Part model, mm, in its own coordinate system. A direction names the side the tool comes from. Coordinates: 2 decimals unless noted, no trailing zeros. Loops run counter-clockwise (first coordinate to the right, second up) from the corner with the lowest first, then second, coordinate; pieces in that order, holes last. Notation, with made-up numbers: (80.5, 9) -> (119.5, 9) arc R17 cw to (119.5, 34) -> close; hole circle Ø11 at (46.25, -7.75). An arc over 180 degrees is marked (long way). Use one line per item in the form item = value. Start each with the question number.
(1) Band-saw the part on D-D on z = 15. Give the cut face in (x, y).
(2) Drill centre lines: L1, parallel to X at y = 5.5, z = 0; L2, parallel to X at y = -0.8, z = 0 (3 decimals); L3, parallel to Y at x = 0, z = -6.5. Where is each one in solid material? Low to high. Write a range as [from, to].
(3) Band-saw the part on C-C on y = 1.75. Give the cut face in (x, z), then the cut area to 3 significant figures.
(4) Pin check, flat tips, straight feed: P1, Ø6, axis at x = -15, z = 7, coming from the +Y side; P2, Ø6, axis at x = 0, z = 0, coming from the -Y side; P3, Ø3.5, axis at x = 0, z = 0, coming from the +Y side; P4, Ø3, axis at y = 0, z = 11, coming from the +X side. Stop position of each tip, or through.
(5) 3-axis set-ups, long thin cutter, end or side, ignore diameter. For faces 4 (the flat face through (-4, 1, 0)), 5 (the cylindrical face through (18.23, 5.227, -5.387)), 6 (the flat face through (1.5, 0, -0.7)): which of +Z, -Z, +X, -X, +Y, -Y reach the whole face in a straight line?
(6) Mould opens along Z. For faces 1 (the flat face through (-18, 9, 0)), 2 (the cylindrical face through (0.45, 0.49, -1.43)), 3 (the cylindrical face through (-1.352, -1.972, 4.292)) say: +Z half, -Z half, draft (parallel to the pull), parting line (faces both ways), or undercut.
(7) Band-saw the part on B-B on x = 0. Give the cut face in (y, z) (3 decimals), then the cut area to 3 significant figures.
(8) Band-saw the part on A-A on z = 0. Give the cut face in (x, y) (3 decimals), then the cut area to 3 significant figures.
```python
from build123d import *

# Parameters (mm, degrees)
SKETCH1_R           = 20.25
BOSS_EXTRUDE1_DEPTH = 9
SKETCH2_R           = 17.75
CUT_EXTRUDE1_DEPTH  = 8
CIRPATTERN1_COUNT   = 3
SKETCH5_R           = 1.5
CUT_EXTRUDE2_DEPTH  = 8
CIRPATTERN2_COUNT   = 3
SKETCH7_R           = 4.5
BOSS_EXTRUDE3_DEPTH = 4
SKETCH8_R           = 3.265
CUT_EXTRUDE3_DEPTH  = 4


with BuildPart() as part:
    # Sketch1 → Boss-Extrude1 (new body)
    with BuildSketch(Plane(origin=(0, 0, 0), x_dir=(1, 0, 0), z_dir=(0, 1, 0))):
        with Locations(Location((0, 0, 0), (0, 0, 270))):
            Circle(SKETCH1_R)
    extrude(amount=BOSS_EXTRUDE1_DEPTH)

    # Sketch2 → Cut-Extrude1 (cut)
    with BuildSketch(Plane(origin=(0, 9, 0), x_dir=(1, 0, 0), z_dir=(0, 1, 0))):
        with Locations(Location((0, 0, 0), (0, 0, 270))):
            Circle(SKETCH2_R)
    extrude(amount=-CUT_EXTRUDE1_DEPTH, mode=Mode.SUBTRACT)

    # Sketch4 → CSK SLOT for M2 Countersunk Flat Head Screw1 (revolve, cut)
    with BuildSketch(Plane(origin=(11.609715894, 0, 11.00974554), x_dir=(0, 0, -1), z_dir=(1, 0, 0))):
        Polygon((0, 0), (0, 6.521032743), (1.2, 5.8), (1.2, 1), (2.2, 0), align=None)
    csk_slot_for_m2_countersunk_flat_head_sc = revolve(axis=Axis((11.609715894, -6.35, 11.00974554), (0, 1, 0)), mode=Mode.SUBTRACT)

    # CirPattern1: CSK SLOT for M2 Countersunk Flat Head Screw1 ×3 about axis
    cirpattern1_axis = Axis((0, 0, 0), (0, 1, 0))
    for i in range(1, CIRPATTERN1_COUNT):
        add(csk_slot_for_m2_countersunk_flat_head_sc.rotate(cirpattern1_axis, i * 360 / CIRPATTERN1_COUNT), mode=Mode.SUBTRACT)

    # Sketch5 → Cut-Extrude2 (cut)
    with BuildSketch(Plane.XZ):
        with Locations(Location((0, 0, 0), (0, 0, 270))):
            Circle(SKETCH5_R)
    extrude(amount=-CUT_EXTRUDE2_DEPTH, mode=Mode.SUBTRACT)

    # Sketch6 → M2 Tapped Hole1 (revolve, cut)
    with BuildSketch(Plane(origin=(-4.560794248, 4.445790719, 19.729715047), x_dir=(0.974306915892993, 0, 0.22522440729877435), z_dir=(0, 1, 0))):
        Polygon((0, 0), (0, 4.980688495), (0.8, 4.5), (0.8, 0), align=None)
    m2_tapped_hole1 = revolve(axis=Axis((-5.990969234, 4.445790719, 25.916563963), (0.22522440729877433, 0, -0.9743069158929931)), mode=Mode.SUBTRACT)

    # CirPattern2: M2 Tapped Hole1 ×3 about axis
    cirpattern2_axis = Axis((0, 9, 0), (0, -1, 0))
    for i in range(1, CIRPATTERN2_COUNT):
        add(m2_tapped_hole1.rotate(cirpattern2_axis, i * 360 / CIRPATTERN2_COUNT), mode=Mode.SUBTRACT)

    # Sketch7 → Boss-Extrude3 (add)
    with BuildSketch(Plane.XZ):
        with Locations(Location((0, 0, 0), (0, 0, 90))):
            Circle(SKETCH7_R)
    extrude(amount=BOSS_EXTRUDE3_DEPTH)

    # Sketch8 → Cut-Extrude3 (cut)
    with BuildSketch(Plane.XZ.offset(4)):
        with Locations(Location((0, 0, 0), (0, 0, 270))):
            Circle(SKETCH8_R)
    extrude(amount=-CUT_EXTRUDE3_DEPTH, mode=Mode.SUBTRACT)


solid = part.part
```
A:
q1.outline = (-13.6, 0) -> (13.6, 0) -> (13.6, 9) -> (9.49, 9) -> (9.49, 1) -> (-9.49, 1) -> (-9.49, 9) -> (-13.6, 9) -> close
q2.L1 = [-20.25, -17.75], [17.75, 20.25]
q2.L2 = [-4.5, -3.265], [3.265, 4.5]
q2.L3 = [0, 1]
q3.outline = circle Ø40.5 at (0, 0); hole circle Ø35.5 at (0, 0)
q3.area = 298 mm²
q4.P1 = 9
q4.P2 = 0
q4.P3 = 1
q4.P4 = 17.88
q5.face_4 = +Y
q5.face_5 = none
q5.face_6 = -Y
q6.face_1 = draft
q6.face_2 = undercut
q6.face_3 = parting line
q7.outline = (-4, -4.5) -> (0, -4.5) -> (0, -20.25) -> (9, -20.25) -> (9, -17.75) -> (1, -17.75) -> (1, -1.5) -> (0, -1.5) -> (0, -3.265) -> (-4, -3.265) -> close; (-4, 3.265) -> (0, 3.265) -> (0, 1.5) -> (1, 1.5) -> (1, 17.75) -> (9, 17.75) -> (9, 20.25) -> (0, 20.25) -> (0, 4.5) -> (-4, 4.5) -> close
q7.area = 87.4 mm²
q8.outline = (-20.25, 0) -> (-4.5, 0) -> (-4.5, -4) -> (-3.265, -4) -> (-3.265, 0) -> (-1.5, 0) -> (-1.5, 1) -> (-17.75, 1) -> (-17.75, 9) -> (-20.25, 9) -> close; (1.5, 0) -> (3.265, 0) -> (3.265, -4) -> (4.5, -4) -> (4.5, 0) -> (20.25, 0) -> (20.25, 9) -> (17.75, 9) -> (17.75, 1) -> (1.5, 1) -> close
q8.area = 87.4 mm²
